Could you check a few things on this model? Use its own coordinates, in mm. Give positions to 0.01 mm unless a question says otherwise; leave off trailing zeros. Write each loop counter-clockwise with the first axis right and the second up, starting at its lowest first coordinate (ties: lowest second). Pieces come first, ordered by that corner, then holes. Notation, with made-up numbers: (32, 57) - (44, 57) arc R32 cw to (44, 87) - close; hole circle Ø3 at (-3.75, 46). An arc over 180 degrees is marked (long way). Answer in a Markdown table with one row per item.
from build123d import *

# Parameters (mm, degrees)
F0_W     = 121.7
F0_H     = 114
F0_R     = 2.5
F0_R_2   = 1.5
F0_R_3   = 11
F0_R_4   = 3.6
F0_R_5   = 4
F1_DEPTH = 7
F2_R     = 2.5
F3_DEPTH = 25


with BuildPart() as f1:
    # F0 (on Front) → F1 (new body)
    with BuildSketch(Plane.XZ):
        with Locations((-56.094777, 36.537357)):
            Rectangle(F0_W, F0_H)
        with Locations((-61.944777, -13.462643)):
            Circle(F0_R, mode=Mode.SUBTRACT)
        with Locations((-107.444777, 21.037357)):
            Circle(F0_R_2, mode=Mode.SUBTRACT)
        with Locations((-91.944777, 36.537357)):
            Circle(F0_R_3, mode=Mode.SUBTRACT)
        with Locations((-76.444777, 21.037357)):
            Circle(F0_R_2, mode=Mode.SUBTRACT)
        with Locations((-61.944777, 16.537357)):
            Circle(F0_R, mode=Mode.SUBTRACT)
        with Locations((-2.244777, -13.462643)):
            Circle(F0_R_4, mode=Mode.SUBTRACT)
        with Locations((-107.444777, 52.037357)):
            Circle(F0_R_2, mode=Mode.SUBTRACT)
        with Locations((-76.444777, 52.037357)):
            Circle(F0_R_2, mode=Mode.SUBTRACT)
        with Locations((-61.944777, 56.537357)):
            Circle(F0_R, mode=Mode.SUBTRACT)
        with Locations((-61.944777, 86.537357)):
            Circle(F0_R, mode=Mode.SUBTRACT)
        with Locations((-2.244777, 86.537357)):
            Circle(F0_R_4, mode=Mode.SUBTRACT)
        with Locations((-91.944777, 36.537357)):
            Circle(F0_R_3)
        with Locations((-91.944777, 36.537357)):
            Circle(F0_R_5, mode=Mode.SUBTRACT)
    extrude(amount=F1_DEPTH)

    # F2 (on face) → F3 (cut)
    with BuildSketch(Plane.XZ.offset(7)):
        with Locations((-35.244777, 46.537357)):
            Circle(F2_R)
        with Locations((-15.244777, 46.537357)):
            Circle(F2_R)
        with Locations((-35.244777, 26.537357)):
            Circle(F2_R)
        with Locations((-15.244777, 26.537357)):
            Circle(F2_R)
    extrude(amount=-F3_DEPTH, mode=Mode.SUBTRACT)


solid = f1.part
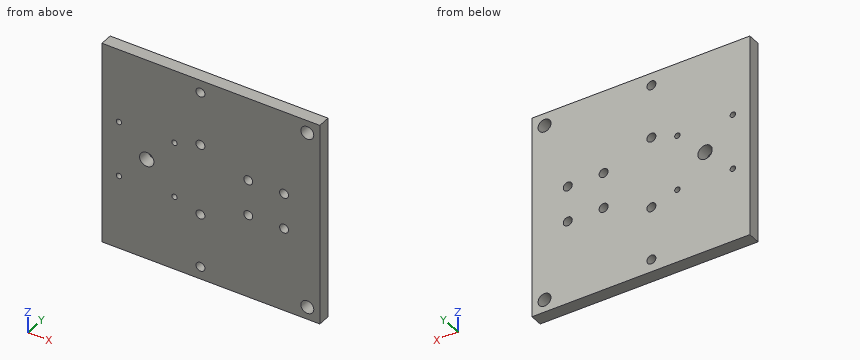
1) If I drill on line 1 (Z direction, x = -34, y = -3); line 2 (Z direction, x = -61.5, y = -4.5); line 3 (X direction, y = -0.75, z = 34), over which ranges is the centre line in solid material (lowest first)?
Check values:
| item | result |
|---|---|
| line 1 | z = -20.46 to 24.37, 28.71 to 44.37, 48.71 to 93.54 |
| line 2 | z = -20.46 to -15.92, -11 to 14.08, 19 to 54.08, 59 to 84.08, 89 to 93.54 |
| line 3 | x = -116.94 to -95.04, -88.85 to 4.76 |
2) Imagine slicing it at A-A (y = -1.25). State how many separate pieces and enclosed holes the cut face has, then the cut area to 3 significant figures.
Check values:
| item | result |
|---|---|
| separate pieces | 1 |
| enclosed holes | 15 |
| area | 13,600 mm2 |
3) Imagine slicing it at B-B (x = -16). List the corners of the cut face in (y, z) for me, then the cut area to 3 significant figures.
Check values:
| item | result |
|---|---|
| outline | (-7, -20.46) - (0, -20.46) - (0, 24.15) - (-7, 24.15) - close; (-7, 28.92) - (0, 28.92) - (0, 44.15) - (-7, 44.15) - close; (-7, 48.92) - (0, 48.92) - (0, 93.54) - (-7, 93.54) - close |
| area | 731 mm2 |
4) Will this pin go through, and if not, where does the flat tip stop? P1, Ø8, axis at x = -61.94, z = 56.54, coming from the +Y side.
Check values:
| item | result |
|---|---|
| P1 | stops at y = 0 |
